Design review of the part built by this model. Coordinates are the model's own, in mm. A direction names the side the tool comes from. Coordinates: 2 decimals unless noted, no trailing zeros.
Q1. Machinability: for faces 1 (the flat face through (-11.47, 8.8, 79.98)), 2 (the flat face through (42.8, 0.11, 53.58)), which of the approach directions +Z, -Z, +X, -X, +Y, -Y give a long, thin tool a straight path to every point of the face, cutting with its end or side? Answer none if there is none.
Q2. Mouldability with a two-part tool opening along Z and no side actions: class faces 3 (the flat face through (-1, 1, 0)), 4 (the cylindrical face through (38.4, -8.47, 46.65)), 5 (the cylindrical face through (-17.34, 78.1, 3.45)) as pulls with the +Z half, pulls with the -Z half, needs draft (parallel to the pull), parting line crosses it, or undercut.
Q3. For probe 1 along Y at (x, z) = (13, 65.5); probe 2 along Z at (x, y) = (17, -73); probe 3 along Z at (x, y) = (-5, -7), list the stretches that pass through material, from the lowest coordinate up.
Q4. Insertion check: pin 1 (1.5 mm diameter, centred on y = -1.5, z = 72.5, fed in from -X); pin 2 (5 mm diameter, centred on x = 38.5, z = 21.5, fed in from +Y); pin 3 (12 mm diameter, centred on x = -52.5, y = 52.5, fed in from -Z); pin 4 (4 mm diameter, centred on x = 40.5, y = 40.5, fed in from +Z). Each pin has a flat end and moves straight along its axis. Give the tip position at first contact, or say it passes through.
Autodesk Fusion 360 part; units mm, degrees
sketch "Skizze1" plane through (0, 0, 0) normal (0, 0, 1) x (1, 0, 0)
  circle A0 centre (0, 0) radius 80
  dimension "d1" = 160
extrude "Extrusion1" add sketch "Skizze1" along normal blind 10
fillet "Abrundung1" radius 3 1 edges at (-74.5862, -28.9292, 10)
sketch "Skizze2" plane through (0, 0, 0) normal (0, 1, 0) x (1, 0, 0)
  line L0 (0, 0) -> (50, 0) construction
  line L1 (50, 0) -> (50, -40) construction
  line L2 (50, -40) -> (0, -40) construction
  line L3 (0, -40) -> (0, 0) construction
  line L4 (50, 0) -> (0, -86.6025) construction
  line L5 (50, 0) -> (160, 0) construction
  line L6 (0, -86.6025) -> (19.9186, -98.1025)
  line L7 (0, -86.6025) -> (23, -86.6025) construction
  line L8 (0, -86.6025) -> (-19.9186, -75.1025)
  dimension "d6" = 50
  dimension "d7" = 40
  dimension "d8" = 120
  dimension "d9" = 100
  dimension "d10" = 30
  dimension "d11" = 23
sketch "Skizze3" plane through (0, 0, 0) normal (1, 0, 0) x (0, 1, 0)
  line L0 (0, 86.6025) -> (0, 75.1025)
  line L1 (0, 86.6025) -> (0, 98.1025)
  line L2 (0, 86.6025) -> (-23, 86.6025)
  line L3 (0, 86.6025) -> (23, 86.6025)
  point P0 (0, 75.1025)
  point P1 (0, 86.6025)
  dimension "d12" = 23
  dimension "d13" = 23
ref_plane "Arbeitsebene1" through (0, 0, 86.6025) normal (0.5, 0, -0.866) x (0, 1, 0)
sketch "Skizze4" plane through (-37.5, 0, 64.9519) normal (0.5, 0, -0.866) x (0, 1, 0)
  line L0 (0, 43.3013) -> (23, 43.3013)
  line L1 (0, 43.3013) -> (-23, 43.3013)
  line L2 (0, 43.3013) -> (0, 20.3013)
  line L3 (0, 43.3013) -> (0, 66.3013)
  circle A0 centre (0, 43.3013) radius 23
  circle A1 centre (0, 43.3013) radius 15.75
  circle A2 centre (0, 43.3013) radius 20
  point P0 (23, 43.3013)
  point P1 (0, 20.3013)
  point P2 (-23, 43.3013)
  point P3 (0, 66.3013)
  point P4 (0, 43.3013)
  dimension "d15" = 46
  dimension "d20" = 31.5
  dimension "d21" = 40
extrude "Extrusion2" add sketch "Skizze4" along normal blind 120
fillet "Abrundung2" radius 15 1 edges at (17.6684, 0, 10)
sketch "Skizze5" plane through (-37.5, 0, 64.9519) normal (-0.5, 0, 0.866) x (0, -1, 0)
  circle A0 centre (0, 43.3013) radius 23
  circle A1 centre (0, 43.3013) radius 15.75
  dimension "d22" = 31.5
extrude "Extrusion3" cut sketch "Skizze5" against normal blind 170 contours A1
sketch "Skizze6" plane through (-37.5, 0, 64.9519) normal (-0.5, 0, 0.866) x (0, -1, 0)
  circle A0 centre (0, 43.3013) radius 15.75
  circle A1 centre (0, 43.3013) radius 23
  circle A2 centre (0, 43.3013) radius 20
  dimension "d25" = 40
extrude "Extrusion4" cut sketch "Skizze6" against normal blind 50 contours A1
sketch "Skizze7" plane through (0, 0, 0) normal (0, 0, 1) x (1, 0, 0)
  line L0 (-80, 80) -> (111.2852, 80)
  line L1 (111.2852, 80) -> (111.2852, -85.555)
  line L2 (111.2852, -85.555) -> (-80, -85.555)
  line L3 (-80, -85.555) -> (-80, 80)
extrude "Extrusion5" cut sketch "Skizze7" against normal blind 90
Response:
1. face 1: +Z, -X, +Y, -Y
1. face 2: none
2. face 3: pulls with the -Z half
2. face 4: undercut
2. face 5: needs draft
3. probe 1: y = -19.99 to -15.73, 15.73 to 19.99
3. probe 2: z = 0 to 10
3. probe 3: z = 0 to 10.2, 57.79 to 67.04
4. pin 1: stops at x = -15.32
4. pin 2: stops at y = 24.11
4. pin 3: stops at z = 0
4. pin 4: stops at z = 10
